from build123d import *

# Parameters (mm, degrees)
SALIENTE_EXTRUIR1_DEPTH = 5.9535
CROQUIS2_R              = 3.969
CORTAR_EXTRUIR1_DEPTH   = 5
MATRIZC1_COUNT          = 3


with BuildPart() as part:
    # Croquis1 → Saliente-Extruir1 (new body, symmetric)
    with BuildSketch(Plane(origin=(0, 0, 0), x_dir=(1, 0, 0), z_dir=(0, 1, 0))):
        Polygon((-2.5, 40.9535), (2.5, 40.9535), (2.5, 1.443375673), (36.716771374, -18.311686491), (34.216771374, -22.641813509), (0, -2.886751346), (-34.216771374, -22.641813509), (-36.716771374, -18.311686491), (-2.5, 1.443375673), align=None)
    extrude(amount=SALIENTE_EXTRUIR1_DEPTH, both=True)

    # Croquis2 → Cortar-Extruir1 (cut)
    with BuildSketch(Plane(origin=(-1.25, 0, 2.165063509), x_dir=(0.866025404, 0, 0.5), z_dir=(-0.5, 0, 0.866025404))):
        with Locations((33.0155, 0)):
            Circle(CROQUIS2_R)
    cortar_extruir1 = extrude(amount=-CORTAR_EXTRUIR1_DEPTH, mode=Mode.SUBTRACT)

    # MatrizC1: Cortar-Extruir1 ×3 about axis
    matrizc1_axis = Axis((0, 5.9535, 0), (0, 1, 0))
    for i in range(1, MATRIZC1_COUNT):
        add(cortar_extruir1.rotate(matrizc1_axis, i * 360 / MATRIZC1_COUNT), mode=Mode.SUBTRACT)


solid = part.part
CAD build for the part. Positions are in the model's coordinates, mm. A direction names the side the tool comes from. Round coordinates to 2 decimals unless told otherwise and drop trailing zeros. Loops run counter-clockwise (first coordinate to the right, second up) from the corner with the lowest first, then second, coordinate; pieces in that order, holes last. Notation, with made-up numbers: (-8, 60) - (-4, 60) arc R32 ccw to (-4, 98) - close; hole circle Ø9 at (35.25, 61). An arc over 180 degrees is marked (long way). Put each result on its own line as item: value.
1. Two-plate mould, pull along Y, no slides. Class faces 5 (the flat face through (-16.869, 0.083, 12.626)), 6 (the cylindrical face through (-26.076, 2.682, 15.015)), 7 (the flat face through (0, -5.954, 2)): released by +Y, released by -Y, zero draft, split by the parting line, or undercut.
Geometry check:
face 5: zero draft
face 6: undercut
face 7: released by -Y
2. Slice it at B-B on y = 0. List the corners of the cut face in (x, z) (1 decimal).
Geometry check:
outline: (-36.7, 18.3) - (-33.3, 16.3) - (-30.8, 20.7) - (-34.2, 22.6) - close; (-26.4, 12.4) - (-2.5, -1.4) - (-2.5, -29) - (2.5, -29) - (2.5, -1.4) - (26.4, 12.4) - (23.9, 16.7) - (0, 2.9) - (-23.9, 16.7) - close; (-2.5, -41) - (2.5, -41) - (2.5, -37) - (-2.5, -37) - close; (30.8, 20.7) - (33.3, 16.3) - (36.7, 18.3) - (34.2, 22.6) - close
3. 3-axis set-ups, long thin cutter, end or side, ignore diameter. For faces 1 (the flat face through (0, 0, -40.954)), 2 (the flat face through (17.348, 0.083, 12.903)), 3 (the flat face through (-2.5, 0, -21)), 4 (the flat face through (2.5, 0, -21)): which of +Z, -Z, +X, -X, +Y, -Y reach the whole face in a straight line?
Geometry check:
face 1: -Z, +X, -X, +Y, -Y
face 2: +Z, +Y, -Y
face 3: -Z, -X, +Y, -Y
face 4: -Z, +X, +Y, -Y
4. Wall check: line 1 (Y direction, x = -28, z = 17.5); line 2 (X direction, y = -1.75, z = -21); line 3 (X direction, y = 2, z = 8). Give the ranges that are in metal, low to high.
Geometry check:
line 1: -5.95 to -3.97, 3.97 to 5.95
line 2: -2.5 to 2.5
line 3: -18.86 to -8.86, 8.86 to 18.86
5. Slice it at A-A on z = 10. List the corners of the cut face in (x, y), and give its area (3 significant figures).
Geometry check:
outline: (-22.32, -5.95) - (-12.32, -5.95) - (-12.32, 5.95) - (-22.32, 5.95) - close; (12.32, -5.95) - (22.32, -5.95) - (22.32, 5.95) - (12.32, 5.95) - close
area: 238 mm²
6. Pin check, flat tips, straight feed: P1, Ø6, axis at y = 3, z = 1, coming from the -X side; P2, Ø4, axis at y = 1.5, z = -1.5, coming from the -X side; P3, Ø4, axis at y = 0.5, z = 10, coming from the +X side. Stop position of each tip, or through.
Geometry check:
P1: x = -11.93
P2: x = -5.87
P3: x = 25.78
7. Slice it at D-D on z = -31. List the corners of the cut face in (x, y), and give its area (3 significant figures).
Geometry check:
outline: (-2.5, -5.95) - (2.5, -5.95) - (2.5, -3.42) - (-2.5, -3.42) - close; (-2.5, 3.42) - (2.5, 3.42) - (2.5, 5.95) - (-2.5, 5.95) - close
area: 25.3 mm²
8. Slice it at C-C on z = -14.5. List the corners of the cut face in (x, y), and give its area (3 significant figures).
Geometry check:
outline: (-2.5, -5.95) - (2.5, -5.95) - (2.5, 5.95) - (-2.5, 5.95) - close
area: 59.5 mm²
